The listing builds one solid part. Answer for the finished solid, in the listing's coordinates (mm). A direction names the side the tool comes from. Coordinates: 2 decimals unless noted, no trailing zeros. Order: outer loops, then holes, each group sorted by start corner. A loop starts at its lowest first (then second) coordinate and runs counter-clockwise, first axis right, second up. Notation, with made-up numbers: (76.25, 55) - (121.25, 55) arc R26 cw to (121.25, 85) - close; hole circle Ø3 at (7.5, 18). An arc over 180 degrees is marked (long way). Use a Markdown table: item, result. Add a question column.
Item 1: The part is cut by section C-C, the plane x = -40. Give the vertices of the cut face in (y, z), then the cut area to 3 significant figures.
Item 2: The mould has two halves that part along Z. Classify faces 1 (the cylindrical face through (22.43, 3.04, -9.4)), 2 (the cylindrical face through (-62.993, 2.958, -0.66)), 3 (the flat face through (33, 3, 0)): released by +Z, released by -Z, zero draft, split by the parting line, or undercut.
Item 3: Flat-ended cylindrical pins translate along their axes: P1, Ø3, axis at y = 4, z = -5.5, coming from the -X side; P2, Ø1.5, axis at y = 1.5, z = 22.5, coming from the -X side; P3, Ø2, axis at y = 1.5, z = 17.5, coming from the -X side. Find the tip coordinate at first contact, or state that the pin passes through.
Item 4: For faces 4 (the flat face through (-16, 0, 0)), 5 (the cylindrical face through (-2.43, 3.04, 21.4)), determine the directions among +Z, -Z, +X, -X, +Y, -Y from which every point of the face is accessible in a straight line to the end or side of a thin tool.
Item 5: Find the intervals of material crossed by line 1 along X through (y, z) = (1.6, 0); line 2 along Z through (x, y) = (19.5, 1); line 3 along X through (y, z) = (2.9, -15), in increasing order.
Item 6: The part is cut by section D-D, the plane z = 25. Give the vertices of the cut face in (x, y).
Item 7: The part is cut by section A-A, the plane x = 29. Give the vertices of the cut face in (y, z).
Item 8: The part is cut by section B-B, the plane z = 0. Give the vertices of the cut face in (x, y), then the cut area to 3 significant figures.
from build123d import *

# Parameters (mm, degrees)
EXTRUDE_1_DEPTH     = 6
SKETCH_2_R          = 13
SKETCH_2_R_2        = 1.35
CUT_EXTRUDE_1_DEPTH = 6
CUT_EXTRUDE_2_DEPTH = 6
SKETCH_4_R          = 1.6
CUT_EXTRUDE_3_DEPTH = 6


with BuildPart() as part:
    # 草图1 → 凸台-拉伸1 (new body)
    with BuildSketch(Plane(origin=(0, 0, 0), x_dir=(1, 0, 0), z_dir=(0, 1, 0))):
        with BuildLine():
            Line((-33, -30), (33, -30))
            Line((33, -30), (33, 30))
            Line((33, 30), (-33, 30))
            ThreePointArc((-33, 30), (-63, 0), (-33, -30))
        make_face()
    extrude(amount=EXTRUDE_1_DEPTH)

    # 草图2 → 切除-拉伸1 (cut)
    with BuildSketch(Plane(origin=(0, 6, 0), x_dir=(1, 0, 0), z_dir=(0, 1, 0))):
        with Locations(Location((-33, 0, 0), (0, 0, 270))):
            Circle(SKETCH_2_R)
        with Locations(Location((-53, 0, 0), (0, 0, 270))):
            Circle(SKETCH_2_R_2)
        with Locations(Location((-23, 17.320508076, 0), (0, 0, 270))):
            Circle(SKETCH_2_R_2)
        with Locations(Location((-23, -17.320508076, 0), (0, 0, 270))):
            Circle(SKETCH_2_R_2)
    extrude(amount=-CUT_EXTRUDE_1_DEPTH, mode=Mode.SUBTRACT)

    # 草图3 → 切除-拉伸2 (cut)
    with BuildSketch(Plane(origin=(0, 6, 0), x_dir=(1, 0, 0), z_dir=(0, 1, 0))):
        with BuildLine():
            Line((21, 14), (-1, 14))
            ThreePointArc((-1, 14), (-2.414213562, 14.585786438), (-3, 16))
            Line((-3, 16), (-3, 20))
            ThreePointArc((-3, 20), (-2.414213562, 21.414213562), (-1, 22))
            Line((-1, 22), (21, 22))
            ThreePointArc((21, 22), (22.414213562, 21.414213562), (23, 20))
            Line((23, 20), (23, 16))
            ThreePointArc((23, 16), (22.414213562, 14.585786438), (21, 14))
        make_face()
        with BuildLine():
            Line((23, 4), (23, 8))
            ThreePointArc((23, 8), (22.414213562, 9.414213562), (21, 10))
            Line((21, 10), (-1, 10))
            ThreePointArc((-1, 10), (-2.414213562, 9.414213562), (-3, 8))
            Line((-3, 8), (-3, 4))
            ThreePointArc((-3, 4), (-2.414213562, 2.585786438), (-1, 2))
            Line((-1, 2), (21, 2))
            ThreePointArc((21, 2), (22.414213562, 2.585786438), (23, 4))
        make_face()
        with BuildLine():
            Line((23, -8), (23, -4))
            ThreePointArc((23, -4), (22.414213562, -2.585786438), (21, -2))
            Line((21, -2), (-1, -2))
            ThreePointArc((-1, -2), (-2.414213562, -2.585786438), (-3, -4))
            Line((-3, -4), (-3, -8))
            ThreePointArc((-3, -8), (-2.414213562, -9.414213562), (-1, -10))
            Line((-1, -10), (21, -10))
            ThreePointArc((21, -10), (22.414213562, -9.414213562), (23, -8))
        make_face()
        with BuildLine():
            Line((23, -20), (23, -16))
            ThreePointArc((23, -16), (22.414213562, -14.585786438), (21, -14))
            Line((21, -14), (-1, -14))
            ThreePointArc((-1, -14), (-2.414213562, -14.585786438), (-3, -16))
            Line((-3, -16), (-3, -20))
            ThreePointArc((-3, -20), (-2.414213562, -21.414213562), (-1, -22))
            Line((-1, -22), (21, -22))
            ThreePointArc((21, -22), (22.414213562, -21.414213562), (23, -20))
        make_face()
    extrude(amount=-CUT_EXTRUDE_2_DEPTH, mode=Mode.SUBTRACT)

    # 草图4 → 切除-拉伸3 (cut)
    with BuildSketch(Plane(origin=(0, 6, 0), x_dir=(1, 0, 0), z_dir=(0, 1, 0))):
        with Locations(Location((29, 25, 0), (0, 0, 270))):
            Circle(SKETCH_4_R)
        with Locations(Location((29, 15, 0), (0, 0, 270))):
            Circle(SKETCH_4_R)
        with Locations(Location((29, -25, 0), (0, 0, 270))):
            Circle(SKETCH_4_R)
        with Locations(Location((29, -15, 0), (0, 0, 270))):
            Circle(SKETCH_4_R)
    extrude(amount=-CUT_EXTRUDE_3_DEPTH, mode=Mode.SUBTRACT)


solid = part.part
Solution:
| question | item | result |
|---|---|---|
| 1 | outline | (0, -29.17) - (6, -29.17) - (6, -10.95) - (0, -10.95) - close; (0, 10.95) - (6, 10.95) - (6, 29.17) - (0, 29.17) - close |
| 1 | area | 219 mm2 |
| 2 | face 1 | undercut |
| 2 | face 2 | split by the parting line |
| 2 | face 3 | zero draft |
| 3 | P1 | stops at x = -62.73 |
| 3 | P2 | stops at x = -53.66 |
| 3 | P3 | stops at x = -58.05 |
| 4 | face 4 | +Z, -Z, +X, -X, -Y |
| 4 | face 5 | +Y, -Y |
| 5 | line 1 | x = -63 to -54.35, -51.65 to -46, -20 to 33 |
| 5 | line 2 | z = -30 to -22, -14 to -10, -2 to 2, 10 to 14, 22 to 30 |
| 5 | line 3 | x = -58.98 to -2.73, 22.73 to 27.4, 30.6 to 33 |
| 6 | outline | (-49.58, 0) - (27.4, 0) - (27.4, 6) - (-49.58, 6) - close; (30.6, 0) - (33, 0) - (33, 6) - (30.6, 6) - close |
| 7 | outline | (0, -30) - (6, -30) - (6, -26.6) - (0, -26.6) - close; (0, -23.4) - (6, -23.4) - (6, -16.6) - (0, -16.6) - close; (0, -13.4) - (6, -13.4) - (6, 13.4) - (0, 13.4) - close; (0, 16.6) - (6, 16.6) - (6, 23.4) - (0, 23.4) - close; (0, 26.6) - (6, 26.6) - (6, 30) - (0, 30) - close |
| 8 | outline | (-63, 0) - (-54.35, 0) - (-54.35, 6) - (-63, 6) - close; (-51.65, 0) - (-46, 0) - (-46, 6) - (-51.65, 6) - close; (-20, 0) - (33, 0) - (33, 6) - (-20, 6) - close |
| 8 | area | 404 mm2 |
